```python
from build123d import *

# Parameters (mm, degrees)
SKETCH_2_R          = 1.520000009
SKETCH_2_R_2        = 1.519999991
SKETCH_2_R_3        = 1.520000003
SKETCH_2_R_4        = 1.519999997
EXTRUDE_3_DEPTH     = 3.5
SKETCH_4_R          = 1.52
CUT_EXTRUDE_2_DEPTH = 59


with BuildPart() as part:
    # 草图2 → 凸台-拉伸3 (new body)
    with BuildSketch(Plane(origin=(0, 0, 0), x_dir=(1, 0, 0), z_dir=(0, 1, 0))):
        with BuildLine():
            ThreePointArc((-11.441254589, -132.131794893), (14.330726674, -93.804971939), (52.669453823, -68.050702844))
            ThreePointArc((52.669453823, -68.050702844), (66.860009927, -29.340594642), (52.82507606, 9.426208049))
            ThreePointArc((52.82507606, 9.426208049), (14.498253105, 35.198189312), (-11.25601599, 73.536916461))
            ThreePointArc((-11.25601599, 73.536916461), (-50.087090736, 87.727594053), (-88.918165482, 73.536916461))
            ThreePointArc((-88.918165482, 73.536916461), (-114.672434576, 35.198189312), (-152.999257531, 9.426208049))
            ThreePointArc((-152.999257531, 9.426208049), (-167.034191399, -29.340594642), (-152.843635295, -68.050702844))
            ThreePointArc((-152.843635295, -68.050702844), (-114.504908145, -93.804971939), (-88.732926883, -132.131794893))
            ThreePointArc((-88.732926883, -132.131794893), (-50.087090736, -146.166850249), (-11.441254589, -132.131794893))
        make_face()
        with Locations((-106.810701812, -85.943239174)):
            Circle(SKETCH_2_R, mode=Mode.SUBTRACT)
        with Locations((-70.087090736, -121.269794335)):
            Circle(SKETCH_2_R, mode=Mode.SUBTRACT)
        with Locations((-80.087090736, -85.943239174)):
            Circle(SKETCH_2_R, mode=Mode.SUBTRACT)
        with Locations((-106.810701812, -59.219628098)):
            Circle(SKETCH_2_R, mode=Mode.SUBTRACT)
        with Locations((-142.137256973, -49.219628098)):
            Circle(SKETCH_2_R, mode=Mode.SUBTRACT)
        with Locations((-50.087090736, -121.269794335)):
            Circle(SKETCH_2_R, mode=Mode.SUBTRACT)
        with Locations((-30.087090736, -121.269794335)):
            Circle(SKETCH_2_R, mode=Mode.SUBTRACT)
        with BuildLine():
            Line((-73.555048946, -95.906459136), (-26.619132526, -95.906459136))
            ThreePointArc((-26.619132526, -95.906459136), (-20.644330739, -101.881260923), (-26.619132526, -107.856062709))
            Line((-26.619132526, -107.856062709), (-73.555048946, -107.856062709))
            ThreePointArc((-73.555048946, -107.856062709), (-79.529850733, -101.881260923), (-73.555048946, -95.906459136))
        make_face(mode=Mode.SUBTRACT)
        with Locations((-50.087090736, -85.943239174)):
            Circle(SKETCH_2_R_2, mode=Mode.SUBTRACT)
        with Locations((-20.087090736, -85.943239174)):
            Circle(SKETCH_2_R, mode=Mode.SUBTRACT)
        with BuildLine():
            Line((10.039848898, -89.354171782), (10.033073964, -89.34738171))
            ThreePointArc((10.033073964, -89.34738171), (10.036665339, -89.34717873), (10.040256701, -89.346975535))
            ThreePointArc((10.040256701, -89.346975535), (10.040052907, -89.350573664), (10.039848898, -89.354171782))
        make_face(mode=Mode.SUBTRACT)
        with Locations((6.63652034, -85.943239174)):
            Circle(SKETCH_2_R, mode=Mode.SUBTRACT)
        with BuildLine():
            ThreePointArc((-82.385679365, -38.265938506), (-91.431989773, -29.219628098), (-82.385679365, -20.17331769))
            Line((-82.385679365, -20.17331769), (-17.788502107, -20.17331769))
            ThreePointArc((-17.788502107, -20.17331769), (-8.742191699, -29.219628098), (-17.788502107, -38.265938506))
            Line((-17.788502107, -38.265938506), (-82.385679365, -38.265938506))
        make_face(mode=Mode.SUBTRACT)
        with Locations((6.63652034, -59.219628098)):
            Circle(SKETCH_2_R_3, mode=Mode.SUBTRACT)
        with Locations((41.963075501, -49.219628098)):
            Circle(SKETCH_2_R_3, mode=Mode.SUBTRACT)
        with Locations((-142.137256973, -29.219628098)):
            Circle(SKETCH_2_R, mode=Mode.SUBTRACT)
        with BuildLine():
            Line((-128.723525347, -52.687586308), (-128.723525347, -5.751669888))
            ThreePointArc((-128.723525347, -5.751669888), (-122.74872356, 0.223131899), (-116.773921774, -5.751669888))
            Line((-116.773921774, -5.751669888), (-116.773921774, -52.687586308))
            ThreePointArc((-116.773921774, -52.687586308), (-122.74872356, -58.662388095), (-128.723525347, -52.687586308))
        make_face(mode=Mode.SUBTRACT)
        with Locations((-142.137256973, -9.219628098)):
            Circle(SKETCH_2_R, mode=Mode.SUBTRACT)
        with Locations((-106.810701812, -29.219628098)):
            Circle(SKETCH_2_R_4, mode=Mode.SUBTRACT)
        with Locations((-106.810701812, 0.780371902)):
            Circle(SKETCH_2_R, mode=Mode.SUBTRACT)
        with Locations((-106.810701812, 27.503982978)):
            Circle(SKETCH_2_R, mode=Mode.SUBTRACT)
        with Locations((-80.087090736, 27.503982978)):
            Circle(SKETCH_2_R, mode=Mode.SUBTRACT)
        with Locations((-70.087090736, 62.830538139)):
            Circle(SKETCH_2_R, mode=Mode.SUBTRACT)
        with Locations((6.63652034, -29.219628098)):
            Circle(SKETCH_2_R_3, mode=Mode.SUBTRACT)
        with BuildLine():
            ThreePointArc((16.599740302, -5.751669888), (22.574542089, 0.223131899), (28.549343876, -5.751669888))
            Line((28.549343876, -5.751669888), (28.549343876, -52.687586308))
            ThreePointArc((28.549343876, -52.687586308), (22.574542089, -58.662388095), (16.599740302, -52.687586308))
            Line((16.599740302, -52.687586308), (16.599740302, -5.751669888))
        make_face(mode=Mode.SUBTRACT)
        with Locations((41.963075501, -29.219628098)):
            Circle(SKETCH_2_R_3, mode=Mode.SUBTRACT)
        with Locations((41.963075501, -9.219628098)):
            Circle(SKETCH_2_R_3, mode=Mode.SUBTRACT)
        with Locations((6.63652034, 0.780371902)):
            Circle(SKETCH_2_R_3, mode=Mode.SUBTRACT)
        with Locations((-50.087090736, 27.503982978)):
            Circle(SKETCH_2_R_4, mode=Mode.SUBTRACT)
        with Locations((-20.087090736, 27.503982978)):
            Circle(SKETCH_2_R, mode=Mode.SUBTRACT)
        with BuildLine():
            Line((-73.555048946, 49.416806513), (-26.619132526, 49.416806513))
            ThreePointArc((-26.619132526, 49.416806513), (-20.644330739, 43.442004727), (-26.619132526, 37.46720294))
            Line((-26.619132526, 37.46720294), (-73.555048946, 37.46720294))
            ThreePointArc((-73.555048946, 37.46720294), (-79.529850733, 43.442004727), (-73.555048946, 49.416806513))
        make_face(mode=Mode.SUBTRACT)
        with Locations((-50.087090736, 62.830538139)):
            Circle(SKETCH_2_R, mode=Mode.SUBTRACT)
        with Locations((-30.087090736, 62.830538139)):
            Circle(SKETCH_2_R, mode=Mode.SUBTRACT)
        with Locations((6.63652034, 27.503982978)):
            Circle(SKETCH_2_R, mode=Mode.SUBTRACT)
    extrude(amount=EXTRUDE_3_DEPTH)

    # 草图4 → 切除-拉伸2 (cut)
    with BuildSketch(Plane.XZ.offset(-7.25)):
        with Locations((-68.087090727, 5.219628098)):
            Circle(SKETCH_4_R)
        with Locations((-32.087090727, 5.219628098)):
            Circle(SKETCH_4_R)
        with Locations((-68.087090727, 53.219628098)):
            Circle(SKETCH_4_R)
        with Locations((-32.087090727, 53.219628098)):
            Circle(SKETCH_4_R)
    extrude(amount=CUT_EXTRUDE_2_DEPTH, mode=Mode.SUBTRACT)


solid = part.part
```
Source: CAD feature listing. Evaluate the final solid. Frame: model axes, mm. A direction names the side the tool comes from. Give positions to 0.01 mm unless a question says otherwise; leave off trailing zeros. Order: outer loops, then holes, each group sorted by start corner. A loop starts at its lowest first (then second) coordinate and runs counter-clockwise, first axis right, second up. Notation, with made-up numbers: (8.25, -32.5) -> (64.25, -32.5) arc R25 cw to (64.25, -3.5) -> close; hole circle Ø10 at (80, -5). An arc over 180 degrees is marked (long way). Use a Markdown table: item, result.
Q1. Section C-C (z = 104). Return the cut outline in (x, y), and give its area (3 significant figures).
A:
| item | result |
|---|---|
| outline | (-105.41, 0) -> (-79.14, 0) -> (-79.14, 3.5) -> (-105.41, 3.5) -> close; (-21.03, 0) -> (5.23, 0) -> (5.23, 3.5) -> (-21.03, 3.5) -> close |
| area | 184 mm^2 |
Q2. Material intervals for line 1 (Z direction, x = -48, y = 3.2); line 2 (X direction, y = 1.75, z = 5); line 3 (X direction, y = 0.25, z = 35.5), sorted ascending. Write a range as [from, to].
A:
| item | result |
|---|---|
| line 1 | [-87.69, -49.42], [-37.47, 20.17], [38.27, 95.91], [107.86, 146.13] |
| line 2 | [-161.95, -128.68], [-116.82, -69.59], [-66.58, -33.59], [-30.58, 16.65], [28.5, 61.78] |
| line 3 | [-166.71, -128.72], [-116.77, -88.9], [-11.28, 16.6], [28.55, 66.53] |
Q3. Section A-A (x = -62.5). Return the cut outline in (y, z), and give its area (3 significant figures).
A:
| item | result |
|---|---|
| outline | (0, -86.43) -> (3.5, -86.43) -> (3.5, -49.42) -> (0, -49.42) -> close; (0, -37.47) -> (3.5, -37.47) -> (3.5, 20.17) -> (0, 20.17) -> close; (0, 38.27) -> (3.5, 38.27) -> (3.5, 95.91) -> (0, 95.91) -> close; (0, 107.86) -> (3.5, 107.86) -> (3.5, 144.87) -> (0, 144.87) -> close |
| area | 663 mm^2 |
Q4. Pull-direction query (X, two-part tool) for faces 1 (the face through (-122.88, 1.73, -0.22)), 2 (the face through (13.87, 1.73, 94.27)), 3 (the face through (-8.744, 1.726, 29.021)), 4 (the face through (-52, 3.5, 2)); classes: +X half, -X half, draft (parallel to the pull), parting line (faces both ways), or undercut.
A:
| item | result |
|---|---|
| face 1 | undercut |
| face 2 | +X half |
| face 3 | undercut |
| face 4 | draft |
Q5. Section B-B (x = 20.5). Return the cut outline in (y, z), and give its area (3 significant figures).
A:
| item | result |
|---|---|
| outline | (0, -29.59) -> (3.5, -29.59) -> (3.5, 0.15) -> (0, 0.15) -> close; (0, 58.29) -> (3.5, 58.29) -> (3.5, 88.06) -> (0, 88.06) -> close |
| area | 208 mm^2 |
Q6. First-contact query: P1, Ø2.5, axis at x = -106.81, z = 29.22, coming from the -Y side; P2, Ø3.5, axis at x = -106.81, z = -27.5, coming from the +Y side; P3, Ø1.8, axis at x = -45, y = 2.5, coming from the -Z side; P4, Ø1.5, axis at y = 2.5, z = 99.5, coming from the -X side. Flat tips, straight axial feed; report the tip coordinate or a pass-through.
A:
| item | result |
|---|---|
| P1 | through |
| P2 | y = 3.5 |
| P3 | z = -87.58 |
| P4 | x = -109.83 |
Q7. Access query for faces 5 (the face through (-122.62, 1.73, 58.66)), 6 (the face through (-49.496, 1.726, -87.725)). Directions: +Z, -Z, +X, -X, +Y, -Y. A direction counts if a zero-diameter tool reaches every point of the face in a straight line with its end or side. Return the directions, or none.
A:
| item | result |
|---|---|
| face 5 | +Y, -Y |
| face 6 | -Z, +Y, -Y |
